Geometry check sheet. Reference: the model listing, model coordinates, mm. A direction names the side the tool comes from. Round coordinates to 2 decimals unless told otherwise and drop trailing zeros. Order: outer loops, then holes, each group sorted by start corner. A loop starts at its lowest first (then second) coordinate and runs counter-clockwise, first axis right, second up. Notation, with made-up numbers: (73.25, -22.5) -> (111.25, -22.5) arc R6 ccw to (111.25, -15.5) -> close; hole circle Ø3 at (33.5, 47.25). An arc over 180 degrees is marked (long way). Answer as a JSON object with one key per item and string values. Group by question number.
from build123d import *

# Parameters (mm, degrees)
BOSS_EXTRUDE1_DEPTH     = 17
CUT_EXTRUDE1_DEPTH      = 41.517773878
CUT_EXTRUDE1_DEPTH_BACK = 41.517773878
SKETCH2_R               = 12.8
SKETCH3_R               = 1.8
CUT_EXTRUDE2_DEPTH      = 28.5
SKETCH4_R               = 3.25
CUT_EXTRUDE3_DEPTH      = 15.3
SKETCH5_R               = 12.85
CUT_EXTRUDE4_DEPTH      = 14
CUT_EXTRUDE5_DEPTH      = 41.517774047
CUT_EXTRUDE5_DEPTH_BACK = 41.517774047
SKETCH6_R               = 1.8
SKETCH7_R               = 3.75
CUT_EXTRUDE6_DEPTH      = 4
CUT_EXTRUDE7_DEPTH      = 4.3


with BuildPart() as part:
    # Sketch1 → Boss-Extrude1 (new, symmetric)
    with BuildSketch(Plane(origin=(0, 0, 0), x_dir=(0, 0, -1), z_dir=(1, 0, 0))):
        with BuildLine():
            Line((-19, -28.7), (19, -28.7))
            ThreePointArc((19, -28.7), (21.828427125, -27.528427125), (23, -24.7))
            Line((23, -24.7), (23, -4.6))
            ThreePointArc((23, -4.6), (21.828427125, -1.771572875), (19, -0.6))
            Line((19, -0.6), (-19, -0.6))
            ThreePointArc((-19, -0.6), (-21.828427125, -1.771572875), (-23, -4.6))
            Line((-23, -4.6), (-23, -24.7))
            ThreePointArc((-23, -24.7), (-21.828427125, -27.528427125), (-19, -28.7))
        make_face()
    extrude(amount=BOSS_EXTRUDE1_DEPTH, both=True)

    # Sketch2 → Cut-Extrude1 (cut, two sides: drawn at the far end of the back side and taken through both)
    with BuildSketch(Plane(origin=(0, 0, 0), x_dir=(0, 0, -1), z_dir=(1, 0, 0)).offset(-CUT_EXTRUDE1_DEPTH_BACK)):
        Circle(SKETCH2_R)
    extrude(amount=CUT_EXTRUDE1_DEPTH + CUT_EXTRUDE1_DEPTH_BACK, mode=Mode.SUBTRACT)

    # Sketch3 → Cut-Extrude2 (cut)
    with BuildSketch(Plane(origin=(0, -28.7, 0), x_dir=(1, 0, 0), z_dir=(0, 1, 0))):
        with Locations(Location((12, -17.5, 0), (0, 0, 236.442690238))):
            Circle(SKETCH3_R)
        with Locations(Location((12, 17.5, 0), (0, 0, 56.442690238))):
            Circle(SKETCH3_R)
        with Locations(Location((-12, -17.5, 0), (0, 0, 236.442690238))):
            Circle(SKETCH3_R)
        with Locations(Location((-12, 17.5, 0), (0, 0, 56.442690238))):
            Circle(SKETCH3_R)
    extrude(amount=CUT_EXTRUDE2_DEPTH, mode=Mode.SUBTRACT)

    # Sketch4 → Cut-Extrude3 (cut)
    with BuildSketch(Plane(origin=(0, -28.7, 0), x_dir=(1, 0, 0), z_dir=(0, 1, 0))):
        with Locations(Location((12, -17.5, 0), (0, 0, 207.48642625))):
            Circle(SKETCH4_R)
        with Locations(Location((12, 17.5, 0), (0, 0, 27.48642625))):
            Circle(SKETCH4_R)
        with Locations(Location((-12, -17.5, 0), (0, 0, 207.48642625))):
            Circle(SKETCH4_R)
        with Locations(Location((-12, 17.5, 0), (0, 0, 27.48642625))):
            Circle(SKETCH4_R)
    extrude(amount=CUT_EXTRUDE3_DEPTH, mode=Mode.SUBTRACT)

    # Sketch5 → Cut-Extrude4 (cut)
    with BuildSketch(Plane(origin=(0, -28.7, 0), x_dir=(1, 0, 0), z_dir=(0, 1, 0))):
        with Locations(Location((0, 0, 0), (0, 0, 270))):
            Circle(SKETCH5_R)
    extrude(amount=CUT_EXTRUDE4_DEPTH, mode=Mode.SUBTRACT)

    # Sketch6 → Cut-Extrude5 (cut, two sides: drawn at the far end of the back side and taken through both)
    with BuildSketch(Plane(origin=(0, 0, 0), x_dir=(0, 0, -1), z_dir=(1, 0, 0)).offset(-CUT_EXTRUDE5_DEPTH_BACK)):
        with Locations((0, -21.7)):
            Circle(SKETCH6_R)
    extrude(amount=CUT_EXTRUDE5_DEPTH + CUT_EXTRUDE5_DEPTH_BACK, mode=Mode.SUBTRACT)

    # Sketch7 → Cut-Extrude6 (cut)
    with BuildSketch(Plane(origin=(17, 0, 0), x_dir=(0, 0, -1), z_dir=(1, 0, 0))):
        with Locations((0, -21.7)):
            Circle(SKETCH7_R)
    extrude(amount=-CUT_EXTRUDE6_DEPTH, mode=Mode.SUBTRACT)

    # Sketch8 → Cut-Extrude7 (cut)
    with BuildSketch(Plane(origin=(-17, 0, 0), x_dir=(0, 0, -1), z_dir=(1, 0, 0))):
        Polygon((-2.85, -20.054551733), (0, -18.409103466), (2.85, -20.054551733), (2.85, -23.345448267), (0, -24.990896534), (-2.85, -23.345448267), align=None)
    extrude(amount=CUT_EXTRUDE7_DEPTH, mode=Mode.SUBTRACT)


solid = part.part
Item 1: Sectioned sample at A-A, the plane y = -12. Enter the section's corners in (x, z), then the cut area to 3 significant figures.
Item 2: Sectioned sample at D-D, the plane x = 0. Enter the section's corners in (y, z).
Item 3: Sectioned sample at B-B, the plane z = 17.5. Enter the section's corners in (x, y).
Item 4: Sectioned sample at C-C, the plane x = -12. Enter the section's corners in (y, z), then the cut area to 3 significant figures.
Item 5: Thickness scan on L1, parallel to X at y = -16.25, z = 17.5; L2, parallel to X at y = -3.25, z = 17.5; L3, parallel to Z at x = 12, y = -5.25. Record the ranges inside material, lowest first.
Item 6: Mould release check, pull along X, two halves, no side actions. Record for faces 1 (the flat face through (17, -17.6, 0.3)), 2 (the flat face through (0, -14.7, 0)), 3 (the flat face through (-14.88, -24.16, -1.44)): pulls with the +X half, pulls with the -X half, needs draft (parallel to the pull), parting line crosses it, or undercut.
Item 7: Set-up check for faces 4 (the cylindrical face through (0.238, -27.559, -21.797)), 5 (the cylindrical face through (15.028, -17.982, 0.488)), 6 (the flat face through (-14.88, -24.18, 1.405)), 7 (the cylindrical face through (11.5, -7.09, 19.23)), 8 (the cylindrical face through (-11.715, -21.157, -20.737)): record each of +Z, -Z, +X, -X, +Y, -Y from which the full face is reachable in a straight line by a thin tool's end or side.
Item 8: Depth check by flat-ended pin: pin 1 Ø4 at (x, z) = (8.5, -4) entering from +Y; pin 2 Ø4.5 at (x, z) = (-12, -17.5) entering from -Y; pin 3 Ø4 at (y, z) = (-21.7, 0) entering from -X; pin 4 Ø3 at (x, z) = (12, -17.5) entering from +Y. Enter the tip coordinate at first touch or a pass-through.
Result:
{
 "1": {"outline": "(-17, -23) -> (17, -23) -> (17, -4.45) -> (-17, -4.45) -> close; (-17, 4.45) -> (17, 4.45) -> (17, 23) -> (-17, 23) -> close; hole circle Ø3.6 at (-12, -17.5); hole circle Ø3.6 at (-12, 17.5); hole circle Ø3.6 at (12, -17.5); hole circle Ø3.6 at (12, 17.5)", "area": "1,220 mm2"},
 "2": {"outline": "(-28.7, -19) arc R4 ccw to (-24.7, -23) -> (-4.6, -23) arc R4 ccw to (-0.6, -19) -> (-0.6, -12.79) arc R12.8 cw to (-0.6, 12.79) -> (-0.6, 19) arc R4 ccw to (-4.6, 23) -> (-24.7, 23) arc R4 ccw to (-28.7, 19) -> (-28.7, 12.85) -> (-14.7, 12.85) -> (-14.7, -12.85) -> (-28.7, -12.85) -> close"},
 "3": {"outline": "(-17, -28.7) -> (-15.25, -28.7) -> (-15.25, -13.4) -> (-13.8, -13.4) -> (-13.8, -0.6) -> (-17, -0.6) -> close; (-10.2, -13.4) -> (-8.75, -13.4) -> (-8.75, -28.7) -> (8.75, -28.7) -> (8.75, -13.4) -> (10.2, -13.4) -> (10.2, -0.6) -> (-10.2, -0.6) -> close; (13.8, -13.4) -> (15.25, -13.4) -> (15.25, -28.7) -> (17, -28.7) -> (17, -0.6) -> (13.8, -0.6) -> close"},
 "4": {"outline": "(-28.7, -14.25) -> (-13.4, -14.25) -> (-13.4, -15.7) -> (-0.6, -15.7) -> (-0.6, -12.79) arc R12.8 cw to (-0.6, 12.79) -> (-0.6, 15.7) -> (-13.4, 15.7) -> (-13.4, 14.25) -> (-28.7, 14.25) -> (-28.7, 4.6) -> (-14.7, 4.6) -> (-14.7, -4.6) -> (-28.7, -4.6) -> close; (-28.3, -20.75) arc R4 ccw to (-24.7, -23) -> (-4.6, -23) arc R4 ccw to (-0.61, -19.3) -> (-13.4, -19.3) -> (-13.4, -20.75) -> close; (-28.3, 20.75) -> (-13.4, 20.75) -> (-13.4, 19.3) -> (-0.61, 19.3) arc R4 ccw to (-4.6, 23) -> (-24.7, 23) arc R4 ccw to start", "area": "618 mm2"},
 "5": {"L1": "x = -17 to -15.25, -8.75 to 8.75, 15.25 to 17", "L2": "x = -17 to -13.8, -10.2 to 10.2, 13.8 to 17", "L3": "z = -23 to -19.3, -15.7 to -11.67, 11.67 to 15.7, 19.3 to 23"},
 "6": {"face 1": "pulls with the +X half", "face 2": "undercut", "face 3": "needs draft"},
 "7": {"face 4": "-Z, +X, -X, -Y", "face 5": "+X", "face 6": "-X", "face 7": "+Y, -Y", "face 8": "-Y"},
 "8": {"pin 1": "stops at y = -11.31", "pin 2": "stops at y = -13.4", "pin 3": "stops at x = -12.7", "pin 4": "passes through"}
}
